Answer from the drawing. Dimensions are ordinates in mm from the lowest x, y and z of the part. Round coordinates to 2 decimals unless told otherwise and drop trailing zeros. Write each loop counter-clockwise with the first axis right and the second up, starting at its lowest first coordinate (ties: lowest second). Pieces come first, ordered by that corner, then holes. Notation, with made-up numbers: (43.25, 3.5) - (63.25, 3.5) arc R15 ccw to (63.25, 17.5) - close; hole circle Ø1 at (15.25, 85.5). An arc over 180 degrees is marked (long way). Answer as CSV lines item,"result". Start each with the question number.
1) Find section A-A on y = 1.4. Determine the outline of the cut face in (x, z), then the cut area to 3 significant figures.
2) Find section C-C on z = 162. Determine the outline of the cut face in (x, y) (1 decimal), then the cut area to 3 significant figures.
3) Find section D-D on x = 23. Determine the outline of the cut face in (y, z), then the cut area to 3 significant figures.
4) Consider line 1 along X through (y, z) = (3.4, 140); line 2 along Z through (x, y) = (41, 2.2); line 3 along Z through (x, y) = (35, 1.45). Determine where each line is inside the solid, lowest interval first.
5) Find section B-B on x = 49. Determine the outline of the cut face in (y, z) (1 decimal), then the cut area to 3 significant figures.
6) Each of these flat-tipped pins is pushed along its axis until it touches: pin 1 (1 mm diameter, centred on y = 2.5, z = 142.5, fed in from -X); pin 2 (3 mm diameter, centred on x = 23, z = 171.18, fed in from +Y). Where does it stop, or does it pass through?
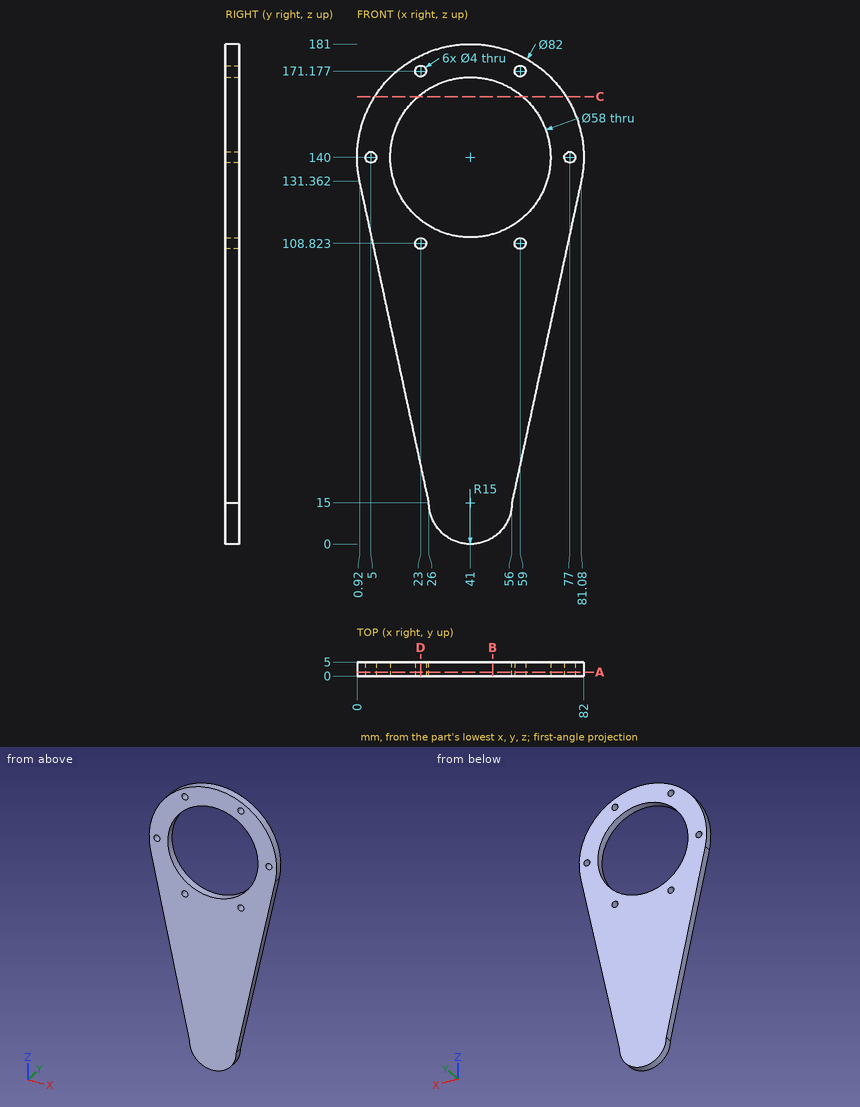
Check values:
1,outline,"(0.92, 131.36) - (26, 15) arc R15 ccw to (56, 15) - (81.08, 131.36) arc R41 ccw (long way) to start; hole circle Ø4 at (5, 140); hole circle Ø58 at (41, 140); hole circle Ø4 at (23, 108.82); hole circle Ø4 at (23, 171.18); hole circle Ø4 at (59, 108.82); hole circle Ø4 at (59, 171.18); hole circle Ø4 at (77, 140)"
1,area,"7,390 mm^2"
2,outline,"(6.4, 0) - (22.1, 0) - (22.1, 5) - (6.4, 5) - close; (59.9, 0) - (75.6, 0) - (75.6, 5) - (59.9, 5) - close"
2,area,"157 mm^2"
3,outline,"(0, 28.92) - (5, 28.92) - (5, 106.82) - (0, 106.82) - close; (0, 110.82) - (5, 110.82) - (5, 117.26) - (0, 117.26) - close; (0, 162.74) - (5, 162.74) - (5, 169.18) - (0, 169.18) - close; (0, 173.18) - (5, 173.18) - (5, 176.84) - (0, 176.84) - close"
3,area,"472 mm^2"
4,line 1,"x = 0 to 3, 7 to 12, 70 to 75, 79 to 82"
4,line 2,"z = 0 to 111, 169 to 181"
4,line 3,"z = 1.25 to 111.63, 168.37 to 180.56"
5,outline,"(0, 2.3) - (5, 2.3) - (5, 112.1) - (0, 112.1) - close; (0, 167.9) - (5, 167.9) - (5, 180.2) - (0, 180.2) - close"
5,area,"611 mm^2"
6,pin 1,"stops at x = 0.05"
6,pin 2,"passes through"
